Can you work these out from the model? Positions are in its coordinate system, mm. Face numbers are marked on the shaded views. A direction names the side the tool comes from. Round coordinates to 2 decimals unless told otherwise and drop trailing zeros. Loops run counter-clockwise (first coordinate to the right, second up) from the corner with the lowest first, then second, coordinate; pieces in that order, holes last.
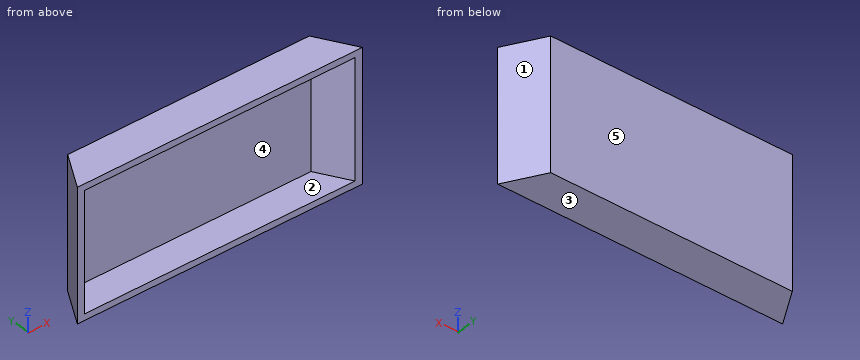
from build123d import *

# Parameters (mm, degrees)
F1_DEPTH = 37.5
F3_DEPTH = 2
F5_DEPTH = 2


with BuildPart() as f1:
    # F0 (on Top) → F1 (new body)
    with BuildSketch(Plane.XY):
        Polygon((-43.273503, -5), (-37.5, 5), (37.5, 5), (43.273503, -5), (45.582904, -5), (38.654701, 7), (-38.654701, 7), (-45.582904, -5), align=None)
    extrude(amount=F1_DEPTH)

    # F2 (on face) → F3 (join)
    with BuildSketch(Plane.XY.offset(37.5)):
        Polygon((-38.654701, 7), (-45.582904, -5), (-43.273503, -5), (-37.5, 5), (37.5, 5), (43.273503, -5), (45.582904, -5), (38.654701, 7), align=None)
        Polygon((-37.5, 5), (-43.273503, -5), (43.273503, -5), (37.5, 5), align=None)
    extrude(amount=F3_DEPTH)

    # F4 (on face) → F5 (join)
    with BuildSketch(Plane(origin=(0, 0, 0), x_dir=(1, 0, 0), z_dir=(0, 0, -1))):
        Polygon((45.582904, 5), (-45.582904, 5), (-38.654701, -7), (38.654701, -7), align=None)
    extrude(amount=F5_DEPTH)


solid = f1.part
(1) If we section it at D-D, the plane y = 3.25: List the corners of the cut face in (x, z) for me.
Worked answers:
outline: (-40.82, -2) - (40.82, -2) - (40.82, 39.5) - (-40.82, 39.5) - close; hole (-38.51, 0) - (38.51, 0) - (38.51, 37.5) - (-38.51, 37.5) - close
(2) If we mould it in two halves opening along Z, with no side actions, what happens to the marked faces 3, 4 and 5? For each: released by +Z, released by -Z, zero draft, split by the parting line, or undercut.
Worked answers:
face 3: released by -Z
face 4: undercut
face 5: zero draft
(3) If we section it at A-A, the plane x = 15.5: List the corners of the cut face in (y, z) for me, then the cut area to 3 significant figures.
Worked answers:
outline: (-5, -2) - (7, -2) - (7, 39.5) - (-5, 39.5) - (-5, 37.5) - (5, 37.5) - (5, 0) - (-5, 0) - close
area: 123 mm2
(4) If we section it at C-C, the plane y = -1.5: List the corners of the cut face in (x, z) for me, then the cut area to 3 significant figures.
Worked answers:
outline: (-43.56, -2) - (43.56, -2) - (43.56, 39.5) - (-43.56, 39.5) - close; hole (-41.25, 0) - (41.25, 0) - (41.25, 37.5) - (-41.25, 37.5) - close
area: 522 mm2
(5) If I drill on line 1 (Z direction, x = 35.5, y = -4); line 2 (Y direction, x = -22.5, z = 16.5); line 3 (X direction, y = 3.5, z = 14), over which ranges is the centre line in solid material (lowest first)?
Worked answers:
line 1: z = -2 to 0, 37.5 to 39.5
line 2: y = 5 to 7
line 3: x = -40.68 to -38.37, 38.37 to 40.68
(6) For the marked faces 1 and 2, which set-ups out of +Z, -Z, +X, -X, +Y, -Y let a thin tool reach every point of the face, with its end or its side?
Worked answers:
face 1: +Z, -Z, +X, +Y
face 2: -Y
(7) If we section it at B-B, the plane z = 8: List the corners of the cut face in (x, y) for me.
Worked answers:
outline: (-45.58, -5) - (-43.27, -5) - (-37.5, 5) - (37.5, 5) - (43.27, -5) - (45.58, -5) - (38.65, 7) - (-38.65, 7) - close
(8) Will these pins go through, and if not, where does the flat tip stop? P1, Ø1.5, axis at x = 26, z = 10, coming from the -Y side; P2, Ø1.5, axis at y = 5.5, z = 17.5, coming from the +X side; P3, Ø2, axis at y = 4, z = 24.5, coming from the +X side.
Worked answers:
P1: stops at y = 5
P2: stops at x = 39.95
P3: stops at x = 40.96
